The listing builds one solid part. Answer for the finished solid, in the listing's coordinates (mm). A direction names the side the tool comes from. Round coordinates to 2 decimals unless told otherwise and drop trailing zeros. Write each loop counter-clockwise with the first axis right and the second up, starting at its lowest first coordinate (ties: lowest second). Pieces come first, ordered by that corner, then holes. Notation, with made-up numbers: (79.5, -3.75) -> (93.5, -3.75) arc R25 ccw to (93.5, 27.25) -> close; hole circle Ø11 at (-6, 52.5). An arc over 180 degrees is marked (long way). Write each question's results on one line, items separated by ' | '. Start each with the question number.
```python
from build123d import *

# Parameters (mm, degrees)
F0_R     = 23.495605
F1_DEPTH = 25.4
F2_R     = 19.972479
F3_DEPTH = 27.178
F4_R     = 16.198988
F5_DEPTH = 37.846
F6_R     = 23.51123
F7_DEPTH = 18.288


with BuildPart() as f1:
    # F0 (on Front) → F1 (new body)
    with BuildSketch(Plane.XZ):
        Circle(F0_R)
    extrude(amount=F1_DEPTH)

    # F2 (on Front) → F3 (cut)
    with BuildSketch(Plane.XZ):
        Circle(F2_R)
    extrude(amount=F3_DEPTH, mode=Mode.SUBTRACT)

    # F4 (on Right) → F5 (cut)
    with BuildSketch(Plane.YZ):
        with Locations((1.37669, 0)):
            Circle(F4_R)
    extrude(amount=F5_DEPTH, mode=Mode.SUBTRACT)

    # F6 (on Front) → F7 (join)
    with BuildSketch(Plane.XZ):
        Circle(F6_R)
    extrude(amount=-F7_DEPTH)


solid = f1.part
```
Q1. The part is cut by section B-B, the plane y = -20. Write down the section's boundary in (x, z).
Q2. Find the intervals of material crossed by line 1 (Z direction, x = 0, y = -5); line 2 (Z direction, x = 5.5, y = -2.5); line 3 (X direction, y = -9.5, z = 0), in increasing order.
Q3. Determine the mould class of faces 1 (the cylindrical face through (20.15, -14.82, 0.34)), 2 (the cylindrical face through (-23.473, -12.522, 1.033)), 3 (the flat face through (0, 18.288, 0)) for opening direction Z: pulls with the +Z half, pulls with the -Z half, needs draft (parallel to the pull), parting line crosses it, or undercut.
Q4. For faces 4 (the cylindrical face through (-18.658, 9.016, -14.306)), 5 (the cylindrical face through (-19.953, -12.522, 0.878)), determine the directions among +Z, -Z, +X, -X, +Y, -Y from which every point of the face is accessible in a straight line to the end or side of a thin tool.
Q5. Each of these flat-tipped pins is pushed along its axis until it touches: pin 1 (6 mm diameter, centred on x = -8.5, y = -6.5, fed in from -Z); pin 2 (2 mm diameter, centred on x = -6.5, y = 2, fed in from +Z); pin 3 (23.5 mm diameter, centred on x = 6.5, z = -1.5, fed in from -Y). Where does it stop, or does it pass through?
Answers follow:
1) outline: circle Ø46.99 at (0, 0); hole circle Ø39.94 at (0, 0)
2) line 1: -23.5 to -19.97, 19.97 to 23.5 | line 2: -22.84 to -19.2, 19.2 to 22.84 | line 3: -23.5 to -19.97
3) face 1: undercut | face 2: parting line crosses it | face 3: needs draft
4) face 4: +Y, -Y | face 5: -Y
5) pin 1: z = -22.84 | pin 2: z = 22.86 | pin 3: y = 0
